Autodesk Inventor part; units mm, degrees
ref_plane "YZ Plane" through (0, 0, 0) normal (1, 0, 0) x (0, 1, 0)
ref_plane "XZ Plane" through (0, 0, 0) normal (0, 1, 0) x (-1, 0, 0)
ref_plane "XY Plane" through (0, 0, 0) normal (0, 0, 1) x (1, 0, 0)
sketch "Sketch1" plane through (0, 0, 0) normal (0, 0, 1) x (1, 0, 0)
  line L0 (13.75, -9.25) -> (-13.75, -9.25)
  line L1 (-13.75, -9.25) -> (-13.75, 9.25)
  line L2 (-13.75, 9.25) -> (13.75, 9.25)
  line L3 (13.75, 9.25) -> (13.75, -9.25)
  line L4 (13.75, -9.25) -> (-13.75, 9.25) construction
  line L5 (-13.75, -9.25) -> (13.75, 9.25) construction
  line L6 (-18, 0) -> (18, 0) construction
  circle A0 centre (-18, 0) radius 4
  circle A1 centre (18, 0) radius 4
  line L7 (32, -1) -> (-32, -1)
  line L8 (-32, -1) -> (-32, 1)
  line L9 (-32, 1) -> (32, 1)
  line L10 (32, 1) -> (32, -1)
  line L11 (32, -1) -> (-32, 1) construction
  line L12 (-32, -1) -> (32, 1) construction
  line L13 (32, -6.5) -> (-32, -6.5)
  line L14 (-32, -6.5) -> (-32, 6.5)
  line L15 (-32, 6.5) -> (32, 6.5)
  line L16 (32, 6.5) -> (32, -6.5)
  line L17 (32, -6.5) -> (-32, 6.5) construction
  line L18 (-32, -6.5) -> (32, 6.5) construction
  point P0 (0, 0)
  point P1 (-21.873, -1)
  point P2 (-13.75, -6.5)
  point P3 (13.75, -6.5)
  point P4 (21.873, -1)
  point P5 (21.873, 1)
  point P6 (13.75, 6.5)
  point P7 (-13.75, 6.5)
  point P8 (-21.873, 1)
  dimension "d0" = 27.5
  dimension "d1" = 18.5
  dimension "d2" = 8
  dimension "d3" = 8
  dimension "d4" = 36
  dimension "d5" = 64
  dimension "d6" = 2
  dimension "d7" = 13
extrude "Extrusion1" add sketch "Sketch1" along normal blind 6.35
fillet "Fillet1" radius 2 4 edges at (13.75, 9.25, 3.175) (-13.75, 9.25, 3.175) (-13.75, -9.25, 3.175) (13.75, -9.25, 3.175)
fillet "Fillet2" radius 2 4 edges at (-32, 6.5, 3.175) (-32, -6.5, 3.175) (32, 6.5, 3.175) (32, -6.5, 3.175)
fillet "Fillet3" radius 1 4 edges at (-13.75, -6.5, 3.175) (-13.75, 6.5, 3.175) (13.75, 6.5, 3.175) (13.75, -6.5, 3.175)
sketch "Sketch2" plane through (0, 0, 6.35) normal (0, 0, 1) x (1, 0, 0)
  line L0 (10, -5.5) -> (-10, -5.5) construction
  line L1 (-10, -5.5) -> (-10, 5.5) construction
  line L2 (-10, 5.5) -> (10, 5.5) construction
  line L3 (10, 5.5) -> (10, -5.5) construction
  line L4 (10, -5.5) -> (-10, 5.5) construction
  line L5 (-10, -5.5) -> (10, 5.5) construction
  circle A0 centre (-10, 5.5) radius 3 construction
  circle A1 centre (-10, -5.5) radius 3 construction
  circle A2 centre (-10, 5.5) radius 1.65 construction
  line L6 (11.75, 9.25) -> (-11.75, 9.25) construction
  point P0 (0, 0)
  dimension "d13" = 20
  dimension "d14" = 11
  dimension "d22" = 6
  dimension "d23" = 6
  dimension "d25" = 3.3
  dimension "d26" = 2.1
hole "Hole1" at (-10, 5.5, 6.35) at (10, 5.5, 6.35) at (10, -5.5, 6.35) at (-10, -5.5, 6.35) direction (0, 0, -1) diameter 3.3 end through all
properties part number "Printhead Belt Retainer Cap THICK" material "Aluminum 6061"
Input: part model. Units: mm. Frame: model coordinates. A direction names the side the tool comes from. Coordinates: 2 decimals unless noted, no trailing zeros. Write each loop counter-clockwise with the first axis right and the second up, starting at its lowest first coordinate (ties: lowest second). Pieces come first, ordered by that corner, then holes. Notation, with made-up numbers: M 19.5,22.25 L 59.5,22.25 A23 ccw 59.5,44.25 Z; hole C -19,70 d9. An arc over 180 degrees is marked long. Answer as a JSON object with one key per item and string values. Group by question number.
(1) Section A-A on x = 10. Output: boundary loops of the cut face in (y, z).
(2) Mould query, pull axis X, two halves, no side actions, for faces 1 (the face through (0, -9.25, 3)), 2 (the face through (-32, 0, 3)), 3 (the face through (11, -4.19, 3.13)), 4 (the face through (11, 6.81, 3.13)). Classes: pulls with the +X half, pulls with the -X half, needs draft (parallel to the pull), parting line crosses it, or undercut.
(3) Section C-C on x = 25.5. Output: boundary loops of the cut face in (y, z), plus the area to 4 significant figures.
(4) Ray query, line 1 along Y through (x, z) = (-10, 4.25); line 2 along X through (y, z) = (4.5, 3); line 3 along X through (y, z) = (5.5, 5). Return the intervals inside material, ascending. Write a range as [from, to].
(5) Set-up query: faces 5 (the face through (-9, 6.81, 3.13)), 6 (the face through (-22, 6.5, 3)), 7 (the face through (22, 6.5, 3)), 8 (the face through (0, 0, 0)), 9 (the face through (-22, -6.5, 3)). Return all of +Z, -Z, +X, -X, +Y, -Y with unobstructed straight access to the full face (end or side cutting, diameter ignored); none if empty.
(6) Section B-B on y = -5.5. Output: boundary loops of the cut face in (x, z), plus the area to 3 significant figures.
(7) Contact query for flat-ended pins moving along their axis: P1, Ø1.9, axis at x = -23.5, z = 4.5, coming from the +Y side; P2, Ø3, axis at x = -10, y = -5.5, coming from the +Z side; P3, Ø3, axis at x = 25, z = 4, coming from the -Y side. Output: stop coordinate, or through.
(8) Section D-D on z = 5. Give the number of separate pieces and of enclosed holes in the cut face, plus the area to 3 significant figures.
Result set:
{
 "1": {"outline": "M -9.25,0 L -7.15,0 L -7.15,6.35 L -9.25,6.35 Z; M -3.85,0 L 3.85,0 L 3.85,6.35 L -3.85,6.35 Z; M 7.15,0 L 9.25,0 L 9.25,6.35 L 7.15,6.35 Z"},
 "2": {"face 1": "needs draft", "face 2": "pulls with the -X half", "face 3": "undercut", "face 4": "undercut"},
 "3": {"outline": "M -6.5,0 L 6.5,0 L 6.5,6.35 L -6.5,6.35 Z", "area": "82.55 mm2"},
 "4": {"line 1": "y = [-9.25, -7.15], [-3.85, 3.85], [7.15, 9.25]", "line 2": "x = [-32, -11.31], [-8.69, 8.69], [11.31, 32]", "line 3": "x = [-31.73, -11.65], [-8.35, 8.35], [11.65, 31.73]"},
 "5": {"face 5": "+Z, -Z", "face 6": "+Z, -Z, -X, +Y", "face 7": "+Z, -Z, +X, +Y", "face 8": "-Z, +X, -X, +Y, -Y", "face 9": "+Z, -Z, -X, -Y"},
 "6": {"outline": "M -31.73,0 L -11.65,0 L -11.65,6.35 L -31.73,6.35 Z; M -8.35,0 L 8.35,0 L 8.35,6.35 L -8.35,6.35 Z; M 11.65,0 L 31.73,0 L 31.73,6.35 L 11.65,6.35 Z", "area": "361 mm2"},
 "7": {"P1": "stops at y = 6.5", "P2": "passes through", "P3": "stops at y = -6.5"},
 "8": {"separate pieces": "1", "enclosed holes": "4", "area": "943 mm2"}
}
